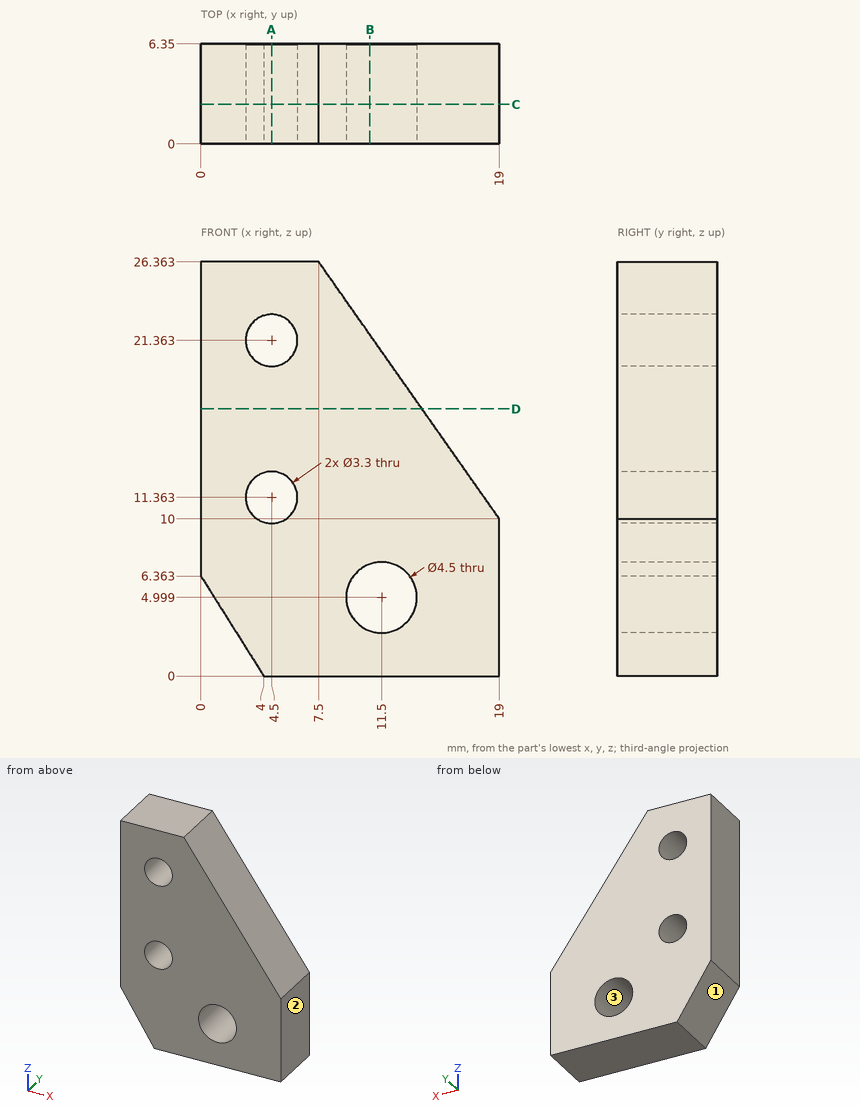
Geometry: see drawing. Coordinates: mm, zero at the bounding-box minimum. Give positions to 0.01 mm unless a question says otherwise; leave off trailing zeros. Order: outer loops, then holes, each group sorted by start corner. A loop starts at its lowest first (then second) coordinate and runs counter-clockwise, first axis right, second up. Notation, with made-up numbers: (16, 39.25) -> (45, 39.25) arc R23 ccw to (45, 62.25) -> close; hole circle Ø3 at (-13, -25). An arc over 180 degrees is marked (long way). Write each question's results on one line, items separated by ' | '. Start each with the question number.
1) Line query: line 1 (Z direction, x = 4.5, y = 3.25); line 2 (Z direction, x = 5.25, y = 5.25) (1 decimal); line 3 (Z direction, x = 11.25, y = 2.25) (1 decimal). Output: solid intervals per line, ascending. Write a range as from..to.
2) Section B-B (x = 10.75). Return loops of the section in (y, z), then the cut area to 3 significant figures.
3) Section C-C (y = 2.5). Return loops of the section in (x, z).
4) First-contact query: pin 1 (5 mm diameter, centred on x = 14, z = 22.5, fed in from +Y); pin 2 (1.5 mm diameter, centred on y = 1.5, z = 23, fed in from +X). Flat tips, straight axial feed; report the tip coordinate or a pass-through.
5) Draft query along Z for the marked faces 1, 2 and 3. Return one class per face: pulls with the +Z half, pulls with the -Z half, needs draft (parallel to the pull), parting line crosses it, or undercut.
6) Section D-D (z = 17). Return loops of the section in (x, y).
7) Section A-A (x = 4.5). Return loops of the section in (y, z).
Calculated:
1) line 1: 0..9.71, 13.01..19.71, 23.01..26.36 | line 2: 0..9.9, 12.8..19.9, 22.8..26.4 | line 3: 0..2.8, 7.2..21
2) outline: (0, 0) -> (6.35, 0) -> (6.35, 2.88) -> (0, 2.88) -> close; (0, 7.12) -> (6.35, 7.12) -> (6.35, 21.74) -> (0, 21.74) -> close | area: 111 mm2
3) outline: (0, 6.36) -> (4, 0) -> (19, 0) -> (19, 10) -> (7.5, 26.36) -> (0, 26.36) -> close; hole circle Ø3.3 at (4.5, 11.36); hole circle Ø3.3 at (4.5, 21.36); hole circle Ø4.5 at (11.5, 5)
4) pin 1: through | pin 2: x = 10.39
5) face 1: pulls with the -Z half | face 2: needs draft | face 3: undercut
6) outline: (0, 0) -> (14.08, 0) -> (14.08, 6.35) -> (0, 6.35) -> close
7) outline: (0, 0) -> (6.35, 0) -> (6.35, 9.71) -> (0, 9.71) -> close; (0, 13.01) -> (6.35, 13.01) -> (6.35, 19.71) -> (0, 19.71) -> close; (0, 23.01) -> (6.35, 23.01) -> (6.35, 26.36) -> (0, 26.36) -> close
